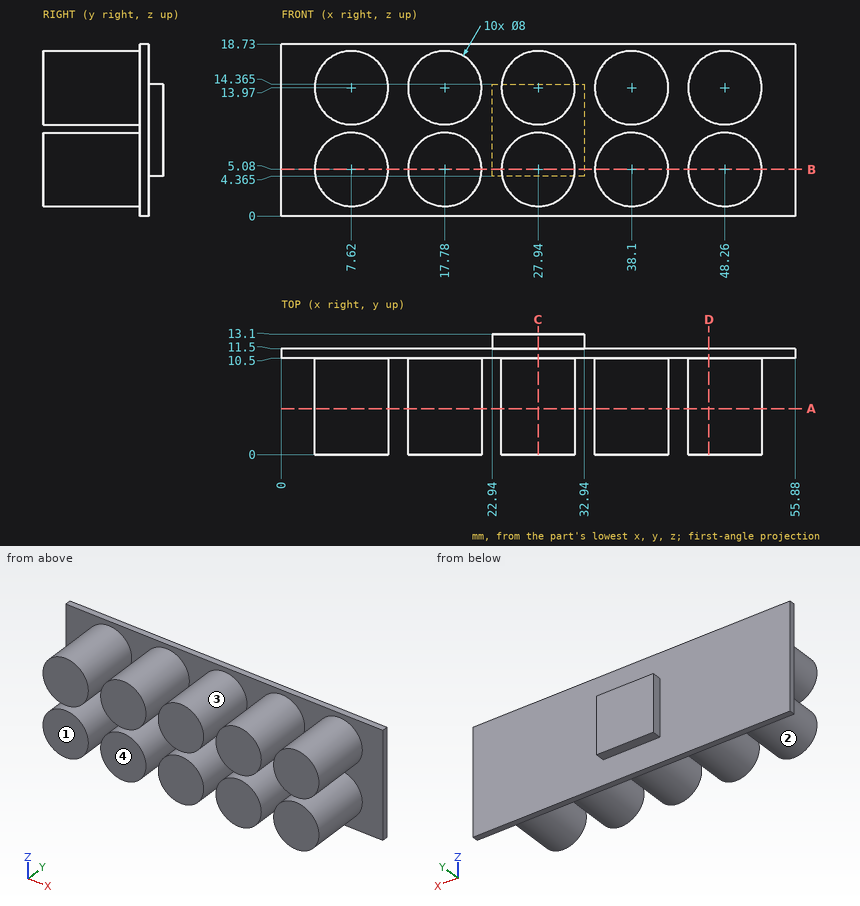
Input: dimensioned drawing with shaded views. Units: mm. Origin: part minimum x, y, z. A direction names the side the tool comes from. Coordinates: 2 decimals unless noted, no trailing zeros. Loops run counter-clockwise (first coordinate to the right, second up) from the corner with the lowest first, then second, coordinate; pieces in that order, holes last. Notation, with made-up numbers: (62, 86) -> (66, 86) arc R13 cw to (66, 97) -> close; hole circle Ø4 at (-4, 23.25). An arc over 180 degrees is marked (long way). One line per item, written item: value. Start each with the question number.
Q1. Contact query for flat-ended pins moving along their axis: P1, Ø3, axis at y = 7.5, z = 9, coming from the -X side; P2, Ø4, axis at x = 21.5, y = 9.5, coming from the +Z side; P3, Ø2, axis at y = 3.5, z = 2, coming from the -X side; P4, Ø5, axis at x = 44, y = 4, coming from the -Z side. Output: stop coordinate, or through.
Q2. Section query B-B, the plane z = 5.08. Return the cut outline in (x, y).
Q3. Set-up query: the marked faces 1 and 2. Return all of +Z, -Z, +X, -X, +Y, -Y with unobstructed straight access to the full face (end or side cutting, diameter ignored); none if empty.
Q4. Section query A-A, the plane y = 5. Give the number of separate pieces and of enclosed holes in the cut face, and give its area (3 significant figures).
Q5. Section query C-C, the plane x = 27.94. Return the cut outline in (y, z) (3 decimals).
Q6. Line query: line 1 along X through (y, z) = (10, 5); line 2 along X through (y, z) = (6.25, 15.75); line 3 along Z through (x, y) = (38, 9). Output: solid intervals per line, ascending.
Q7. Section query D-D, the plane x = 46.5. Return the cut outline in (y, z).
Q8. Mould query, pull axis Z, two halves, no side actions, for the marked faces 3 and 4. Classes: pulls with the +Z half, pulls with the -Z half, needs draft (parallel to the pull), parting line crosses it, or undercut.
Results:
1. P1: x = 4.44
1. P2: z = 18.73
1. P3: x = 4.2
1. P4: z = 1.49
2. outline: (0, 10.5) -> (3.62, 10.5) -> (3.62, 0) -> (11.62, 0) -> (11.62, 10.5) -> (13.78, 10.5) -> (13.78, 0) -> (21.78, 0) -> (21.78, 10.5) -> (23.94, 10.5) -> (23.94, 0) -> (31.94, 0) -> (31.94, 10.5) -> (34.1, 10.5) -> (34.1, 0) -> (42.1, 0) -> (42.1, 10.5) -> (44.26, 10.5) -> (44.26, 0) -> (52.26, 0) -> (52.26, 10.5) -> (55.88, 10.5) -> (55.88, 11.5) -> (32.94, 11.5) -> (32.94, 13.1) -> (22.94, 13.1) -> (22.94, 11.5) -> (0, 11.5) -> close
3. face 1: +Z, -Z, +X, -X, -Y
3. face 2: -Y
4. separate pieces: 10
4. enclosed holes: 0
4. area: 503 mm^2
5. outline: (0, 1.08) -> (10.5, 1.08) -> (10.5, 0) -> (11.5, 0) -> (11.5, 4.365) -> (13.1, 4.365) -> (13.1, 14.365) -> (11.5, 14.365) -> (11.5, 18.73) -> (10.5, 18.73) -> (10.5, 17.97) -> (0, 17.97) -> (0, 9.97) -> (10.5, 9.97) -> (10.5, 9.08) -> (0, 9.08) -> close
6. line 1: 3.62 to 11.62, 13.78 to 21.78, 23.94 to 31.94, 34.1 to 42.1, 44.26 to 52.26
6. line 2: 4.04 to 11.2, 14.2 to 21.36, 24.36 to 31.52, 34.52 to 41.68, 44.68 to 51.84
6. line 3: 1.08 to 9.08, 9.97 to 17.97
7. outline: (0, 1.49) -> (10.5, 1.49) -> (10.5, 0) -> (11.5, 0) -> (11.5, 18.73) -> (10.5, 18.73) -> (10.5, 17.56) -> (0, 17.56) -> (0, 10.38) -> (10.5, 10.38) -> (10.5, 8.67) -> (0, 8.67) -> close
8. face 3: undercut
8. face 4: needs draft
